Autodesk Inventor part; units mm, degrees
ref_plane "YZ Plane" through (0, 0, 0) normal (1, 0, 0) x (0, 1, 0)
ref_plane "XZ Plane" through (0, 0, 0) normal (0, 1, 0) x (-1, 0, 0)
ref_plane "XY Plane" through (0, 0, 0) normal (0, 0, 1) x (1, 0, 0)
sketch "Sketch1" plane through (0, 0, 0) normal (0, 0, 1) x (1, 0, 0)
  line L0 (-101.6, -76.2) -> (101.6, -76.2)
  line L1 (101.6, -76.2) -> (101.6, 76.2)
  line L2 (101.6, 76.2) -> (-101.6, 76.2)
  line L3 (-101.6, 76.2) -> (-101.6, -76.2)
  line L4 (-101.6, -76.2) -> (101.6, 76.2) construction
  line L5 (101.6, -76.2) -> (-101.6, 76.2) construction
  point P0 (0, 0)
  dimension "d0" = 152.4
  dimension "d1" = 203.2
extrude "Extrusion1" add sketch "Sketch1" along normal blind 3.175
fillet "Fillet1" radius 12.7 4 edges at (101.6, 76.2, 1.5875) (101.6, -76.2, 1.5875) (-101.6, -76.2, 1.5875) (-101.6, 76.2, 1.5875)
sketch "Sketch2" plane through (0, 0, 3.175) normal (0, 0, 1) x (1, 0, 0)
  line L0 (101.6, -73.1012) -> (-101.6, -73.1012)
  line L1 (101.6, -73.1012) -> (101.6, -53.8988)
  line L2 (-101.6, -53.8988) -> (101.6, -53.8988)
  line L3 (-97.2058, -18.9992) -> (-97.2058, 44.2468)
  line L4 (-97.2058, -18.9992) -> (-85.1719, -18.9992)
  line L5 (-85.1719, -18.9992) -> (-31.877, 34.2957)
  line L6 (-31.877, 34.2957) -> (-31.877, 46.3296)
  line L7 (-95.123, 46.3296) -> (-31.877, 46.3296)
  line L8 (-101.6, 63.5) -> (-101.6, -63.5)
  line L9 (-88.9, -76.2) -> (88.9, -76.2)
  arc A0 (-97.2058, 44.2468) -> (-95.123, 46.3296) centre (-97.1931, 46.3169) ccw
  circle A1 centre (-74.2399, 4.9487) radius 2.0701
  circle A2 centre (-56.2794, 41.3242) radius 2.4892
  circle A3 centre (-92.2004, 5.4032) radius 2.4892
  circle A4 centre (-74.2399, 23.3637) radius 14.2875
  circle A5 centre (-74.2399, 41.7787) radius 2.0701
  circle A6 centre (-91.7406, 40.8644) radius 3.7211
  circle A7 centre (-55.8249, 23.3637) radius 2.0701
  circle A8 centre (-92.6549, 23.3637) radius 2.0701
  circle A9 centre (-88.9, -63.5) radius 2.0701
  circle A10 centre (-63.5, -63.5) radius 2.0701
  circle A11 centre (-38.1, -63.5) radius 2.0701
  circle A12 centre (-12.7, -63.5) radius 2.0701
  circle A13 centre (12.7, -63.5) radius 2.0701
  circle A14 centre (38.1, -63.5) radius 2.0701
  circle A15 centre (63.5, -63.5) radius 2.0701
  circle A16 centre (88.9, -63.5) radius 2.0701
  arc A17 (65.5687, 63.5) -> (61.4313, 63.5) centre (63.5, 63.4238) ccw
  line L10 (61.4313, 63.5) -> (40.1687, 63.5)
  arc A18 (40.1687, 63.5) -> (36.0313, 63.5) centre (38.1, 63.4238) ccw
  line L11 (36.0313, 63.5) -> (14.7687, 63.5)
  arc A19 (14.7687, 63.5) -> (10.6313, 63.5) centre (12.7, 63.4238) ccw
  line L12 (10.6313, 63.5) -> (-10.6313, 63.5)
  arc A20 (-10.6313, 63.5) -> (-14.7687, 63.5) centre (-12.7, 63.4238) ccw
  line L13 (-14.7687, 63.5) -> (-36.0313, 63.5)
  arc A21 (-36.0313, 63.5) -> (-40.1687, 63.5) centre (-38.1, 63.4238) ccw
  line L14 (-40.1687, 63.5) -> (-61.4313, 63.5)
  arc A22 (-61.4313, 63.5) -> (-65.5687, 63.5) centre (-63.5, 63.4238) ccw
  line L15 (-65.5687, 63.5) -> (-86.8313, 63.5)
  arc A23 (-86.8313, 63.5) -> (-90.9687, 63.5) centre (-88.9, 63.4238) ccw
  line L16 (-90.9687, 63.5) -> (-101.6, 63.5)
  line L17 (-101.6, 76.1238) -> (-101.6, 63.5)
  line L18 (-101.6, 76.1238) -> (101.6, 76.1238)
  line L19 (101.6, 63.5) -> (101.6, 76.1238)
  line L20 (101.6, 63.5) -> (90.9687, 63.5)
  arc A24 (90.9687, 63.5) -> (86.8313, 63.5) centre (88.9, 63.4238) ccw
  line L21 (86.8313, 63.5) -> (65.5687, 63.5)
  line L22 (-101.6, -53.8988) -> (-101.6, -73.1012)
  point P0 (0, 0)
  point P1 (-88.9, -63.5)
  point P2 (-63.5, -63.5)
  point P3 (-38.1, -63.5)
  point P4 (-12.7, -63.5)
  point P5 (12.7, -63.5)
  point P6 (38.1, -63.5)
  point P7 (63.5, -63.5)
  point P8 (88.9, -63.5)
  dimension "d12" = 12.7
  dimension "d13" = 12.7
  dimension "d16" = 25.4
hole "Hole1" at (-63.5, -63.5, 3.175) at (-88.9, -63.5, 3.175) at (-38.1, -63.5, 3.175) at (-12.7, -63.5, 3.175) at (12.7, -63.5, 3.175) at (38.1, -63.5, 3.175) at (63.5, -63.5, 3.175) at (88.9, -63.5, 3.175) at (-88.9, 63.4238, 3.175) at (-63.5, 63.4238, 3.175) at (-38.1, 63.4238, 3.175) at (-12.7, 63.4238, 3.175) at (12.7, 63.4238, 3.175) at (38.1, 63.4238, 3.175) at (63.5, 63.4238, 3.175) at (88.9, 63.4238, 3.175) direction (0, 0, -1) diameter 4.1402 end through all
sketch "Sketch3" plane through (0, 0, 0) normal (0, 0, -1) x (-1, 0, 0)
  line L0 (88.9, -76.2) -> (-88.9, -76.2)
  line L1 (25.4, -76.2) -> (-25.4, -76.2)
  line L2 (-25.4, -76.2) -> (-25.4, -44.45)
  line L3 (-25.4, -44.45) -> (25.4, -44.45)
  line L4 (25.4, -44.45) -> (25.4, -76.2)
  line L5 (101.6, 63.5) -> (101.6, -63.5)
  point P0 (0, 0)
  dimension "d21" = 50.8
  dimension "d22" = 31.75
  dimension "d23" = 76.2
extrude "Extrusion2" cut sketch "Sketch3" against normal through all
fillet "Fillet2" radius 12.7 4 edges at (-25.4, -76.2, 1.5875) (-25.4, -44.45, 1.5875) (25.4, -44.45, 1.5875) (25.4, -76.2, 1.5875)
properties part number "C12_TK_UpperFrameSupport" material "Polycarbonate, Clear"
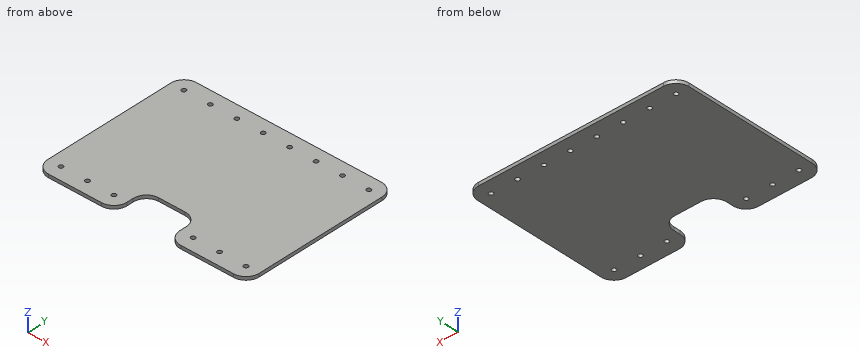
Geometry check sheet. Reference: the model listing, model coordinates, mm. Give positions to 0.01 mm unless a question says otherwise; leave off trailing zeros. Loops run counter-clockwise (first coordinate to the right, second up) from the corner with the lowest first, then second, coordinate; pieces in that order, holes last.
(1) Thickness scan on L1, parallel to Y at x = 88.9, z = 0.7; L2, parallel to Y at x = -12.7, z = 1.25; L3, parallel to Y at x = 89.5, z = 0.2. Record the ranges inside material, lowest first.
From the geometry:
L1: y = -76.2 to -65.57, -61.43 to 61.35, 65.49 to 76.2
L2: y = -44.45 to 61.35, 65.49 to 76.2
L3: y = -76.19 to -65.48, -61.52 to 61.44, 65.41 to 76.19
(2) Section check B-B on z = 1.85. Count the separate pieces of the cut face and the enclosed holes in it, then the cut area to 3 significant figures.
From the geometry:
separate pieces: 1
enclosed holes: 14
area: 29,000 mm2
(3) Section check A-A on x = -63.5. Record the cut outline in (y, z) (3 decimals), then the cut area to 3 significant figures.
From the geometry:
outline: (-76.2, 0) - (-65.57, 0) - (-65.57, 3.175) - (-76.2, 3.175) - close; (-61.43, 0) - (61.354, 0) - (61.354, 3.175) - (-61.43, 3.175) - close; (65.494, 0) - (76.2, 0) - (76.2, 3.175) - (65.494, 3.175) - close
area: 458 mm2
(4) Depth check by flat-ended pin: pin 1 Ø1 at (x, z) = (-2, 1.5) entering from -Y. Enter the tip coordinate at first touch or a pass-through.
From the geometry:
pin 1: stops at y = -44.45
